Can you work these out from the model? Positions are in its coordinate system, mm. Face numbers are marked on the shaded views. A direction names the side the tool comes from. Give positions to 0.01 mm unless a question says otherwise; leave off trailing zeros. Loops run counter-clockwise (first coordinate to the right, second up) from the corner with the lowest first, then second, coordinate; pieces in that order, holes last. Notation, with made-up numbers: (18, -15) -> (22, -15) arc R25 cw to (22, 2) -> close; hole circle Ø9 at (58.5, 75.25). An arc over 180 degrees is marked (long way). Return JSON: item names as keys, results as strings. Group by question number.
Q1. I need wall thicknesses on line 1 along Z through (x, y) = (0, -10); line 2 along X through (y, z) = (-7.5, 43); line 3 along X through (y, z) = (-8.5, -0.5). Which ranges of each line are inside material? Lowest first, please. Write a range as [from, to].
Q2. Which directions (+Z, -Z, +X, -X, +Y, -Y) give clear straight access to the entire face, cutting with the end or side of a thin tool? Please do the marked faces 1, 2 and 3.
Q3. Suppose I cut it at B-B, the plane x = 24. Please give me the cut outline in (y, z), and give its area (3 significant figures).
Q4. Suppose I cut it at C-C, the plane y = -3.75. Count the separate pieces of the cut face and the enclosed holes in it, and give its area (3 significant figures).
Q5. Suppose I cut it at A-A, the plane z = 40.5. Please give me the cut outline in (x, y) (3 decimals).
Q6. Will these pins go through, and if not, where does the flat tip stop? pin 1 (20.5 mm diameter, centred on x = 0, z = 42.86, fed in from -Y); pin 2 (1.5 mm diameter, centred on y = -7, z = -3.5, fed in from -X); pin 3 (2 mm diameter, centred on y = -1.5, z = 13.5, fed in from -X); pin 4 (4 mm diameter, centred on y = -8, z = 26, fed in from -X).
Q7. Suppose I cut it at D-D, the plane x = -5. Please give me the cut outline in (y, z).
Q8. Thinking about a two-plate mould opening in X: for the marked faces 4, 5 and 6, which applies, pulls with the +X half, pulls with the -X half, needs draft (parallel to the pull), parting line crosses it, or undercut?
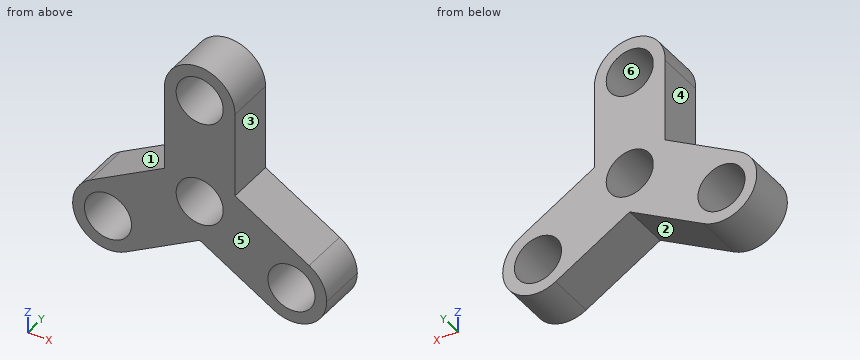
```python
from build123d import *

# Parameters (mm, degrees)
F1_DEPTH = 12.7
F2_R     = 6.35
F3_DEPTH = 12.701


with BuildPart() as f1:
    # F0 (on Front) → F1 (new body)
    with BuildSketch(Plane.XZ):
        with BuildLine():
            ThreePointArc((-9.5140915631, 42.4067734045), (0.2279285655, 33.3402274997), (9.525, 42.8625))
            ThreePointArc((9.525, 42.8625), (-0.2279285655, 52.3847725003), (-9.5140915631, 42.4067734045))
        make_face()
        with BuildLine():
            Line((9.525, 19.786761314), (9.525, 42.8625))
            ThreePointArc((9.525, 42.8625), (0.2279285655, 33.3402274997), (-9.5140915631, 42.4067734045))
            Line((-9.5140915631, 42.4067734045), (-9.5140915631, 19.793059303))
            Line((-9.5140915631, 19.793059303), (-29.5091759131, 8.248891971))
            ThreePointArc((-29.5091759131, 8.248891971), (-19.9841759131, 8.248891971), (-15.2216759131, 0))
            ThreePointArc((-15.2216759131, 0), (-16.4977839421, -4.7625), (-19.9841759131, -8.248891971))
            Line((-19.9841759131, -8.248891971), (0, 3.2889773719))
            Line((0, 3.2889773719), (19.9841759131, -8.248891971))
            ThreePointArc((19.9841759131, -8.248891971), (16.4977839421, 4.7625), (29.5091759131, 8.248891971))
            Line((29.5091759131, 8.248891971), (9.525, 19.786761314))
        make_face()
        with BuildLine():
            ThreePointArc((-15.2216759131, 0), (-19.9841759131, 8.248891971), (-29.5091759131, 8.248891971))
            ThreePointArc((-29.5091759131, 8.248891971), (-32.9955678842, -4.7625), (-19.9841759131, -8.248891971))
            ThreePointArc((-19.9841759131, -8.248891971), (-16.4977839421, -4.7625), (-15.2216759131, 0))
        make_face()
        with BuildLine():
            ThreePointArc((34.2716759131, 0), (32.9955678842, 4.7625), (29.5091759131, 8.248891971))
            ThreePointArc((29.5091759131, 8.248891971), (16.4977839421, 4.7625), (19.9841759131, -8.248891971))
            ThreePointArc((19.9841759131, -8.248891971), (29.5091759131, -8.248891971), (34.2716759131, 0))
        make_face()
    extrude(amount=F1_DEPTH)

    # F2 (on face) → F3 (cut, through all)
    with BuildSketch(Plane.XZ.offset(12.7)):
        with Locations((-24.7466759131, 0)):
            Circle(F2_R)
        with Locations((0, 14.2875)):
            Circle(F2_R)
        with Locations((0, 42.8625)):
            Circle(F2_R)
        with Locations((24.7466759131, 0)):
            Circle(F2_R)
    extrude(amount=-F3_DEPTH, mode=Mode.SUBTRACT)


solid = f1.part
```
Ans:
{
 "1": {"line 1": "z = [3.29, 7.94], [20.64, 36.51], [49.21, 52.39]", "line 2": "x = [-9.52, -6.35], [6.35, 9.52]", "line 3": "x = [-34.26, -31.08], [-18.42, -6.56], [6.56, 18.42], [31.08, 34.26]"},
 "2": {"face 1": "+Z, -X, +Y, -Y", "face 2": "-Z, +Y, -Y", "face 3": "+Z, +X, +Y, -Y"},
 "3": {"outline": "(-12.7, -9.5) -> (0, -9.5) -> (0, -6.31) -> (-12.7, -6.31) -> close; (-12.7, 6.31) -> (0, 6.31) -> (0, 11.43) -> (-12.7, 11.43) -> close", "area": "106 mm^2"},
 "4": {"separate pieces": "1", "enclosed holes": "4", "area": "1,400 mm^2"},
 "5": {"outline": "(-9.514, -12.7) -> (-5.894, -12.7) -> (-5.894, 0) -> (-9.514, 0) -> close; (5.894, -12.7) -> (9.525, -12.7) -> (9.525, 0) -> (5.894, 0) -> close"},
 "6": {"pin 1": "stops at y = -12.7", "pin 2": "stops at x = -33.87", "pin 3": "stops at x = -22.15", "pin 4": "stops at x = -9.51"},
 "7": {"outline": "(-12.7, 0.4) -> (0, 0.4) -> (0, 10.37) -> (-12.7, 10.37) -> close; (-12.7, 18.2) -> (0, 18.2) -> (0, 38.95) -> (-12.7, 38.95) -> close; (-12.7, 46.78) -> (0, 46.78) -> (0, 50.97) -> (-12.7, 50.97) -> close"},
 "8": {"face 4": "pulls with the -X half", "face 5": "needs draft", "face 6": "undercut"}
}
